```python
from build123d import *

# Parameters (mm, degrees)
F0_W     = 180
F0_H     = 40
F1_DEPTH = 22
F3_D     = 22
F3_DEPTH = 15
F3_TIP   = 6.6094668093
F5_D     = 11
F5_DEPTH = 12
F5_TIP   = 3.3047334047
F7_D     = 11
F7_DEPTH = 12
F7_TIP   = 3.3047334047
F9_D     = 11
F9_DEPTH = 12
F9_TIP   = 3.3047334047


with BuildPart() as f1:
    # F0 (on Top) → F1 (new body)
    with BuildSketch(Plane.XY):
        Rectangle(F0_W, F0_H)
    extrude(amount=-F1_DEPTH)

    # F3
    with Locations(Plane.XY):
        with Locations((0, 0)):
            Hole(F3_D / 2, depth=F3_DEPTH)
            with Locations((0, 0, -(F3_DEPTH + F3_TIP / 2))):  # 118° drill point
                Cone(0, F3_D / 2, F3_TIP, mode=Mode.SUBTRACT)

    # F5
    with Locations(Plane(origin=(-90, 0, 0), x_dir=(0, -1, 0), z_dir=(-1, 0, 0))):
        with Locations((0, -11)):
            Hole(F5_D / 2, depth=F5_DEPTH)
            with Locations((0, 0, -(F5_DEPTH + F5_TIP / 2))):  # 118° drill point
                Cone(0, F5_D / 2, F5_TIP, mode=Mode.SUBTRACT)

    # F7
    with Locations(Plane.YZ.offset(90)):
        with Locations((0, -11)):
            Hole(F7_D / 2, depth=F7_DEPTH)
            with Locations((0, 0, -(F7_DEPTH + F7_TIP / 2))):  # 118° drill point
                Cone(0, F7_D / 2, F7_TIP, mode=Mode.SUBTRACT)

    # F9
    with Locations(Plane(origin=(0, 20, 0), x_dir=(-1, 0, 0), z_dir=(0, 1, 0))):
        with Locations((-50, -11)):
            Hole(F9_D / 2, depth=F9_DEPTH)
            with Locations((0, 0, -(F9_DEPTH + F9_TIP / 2))):  # 118° drill point
                Cone(0, F9_D / 2, F9_TIP, mode=Mode.SUBTRACT)


solid = f1.part
```
Verification items for the finished model (mm, model axes). A direction names the side the tool comes from. Round coordinates to 2 decimals unless told otherwise and drop trailing zeros. Answer as a JSON object with one key per item and string values. Group by question number.
Q1. Mould release check, pull along Z, two halves, no side actions. Record for faces 1 (the cylindrical face through (-83.92, -1.19, -16.37)), 2 (the flat face through (-1, 0, -22)), 3 (the conical face through (49.12, 5.27, -11.37)), 4 (the flat face through (-1, 14, 0)): released by +Z, released by -Z, zero draft, split by the parting line, or undercut.
Q2. Tool access check on faces 5 (the cylindrical face through (44.505, 13.916, -10.758)), 6 (the cylindrical face through (83.92, 1.19, -16.37)), 7 (the flat face through (-1, 20, -11)), 8 (the cylindrical face through (2.38, -10.74, -7.6)), 9 (the flat face through (90, -5, -6)). Record the directions out of +Z, -Z, +X, -X, +Y, -Y that give a thin tool (end or side, any length) a straight path to the whole face; none if there is none.
Q3. Thickness scan on line 1 (Z direction, x = -87, y = 0); line 2 (Y direction, x = -84.5, z = -11); line 3 (X direction, y = 9, z = -4.5). Record the ranges inside material, lowest first.
Q4. Go/stop test with flat-tipped pins: pin 1 Ø1.5 at (y, z) = (4, -10.5) entering from -X; pin 2 Ø10 at (y, z) = (0, -11) entering from +X; pin 3 Ø10 at (y, z) = (0, -11) entering from -X. Record where each tip stops, or that it passes through.
Found:
{
 "1": {"face 1": "undercut", "face 2": "released by -Z", "face 3": "undercut", "face 4": "released by +Z"},
 "2": {"face 5": "+Y", "face 6": "+X", "face 7": "+Z, -Z, +X, -X, +Y", "face 8": "+Z", "face 9": "+Z, -Z, +X, +Y, -Y"},
 "3": {"line 1": "z = -22 to -16.5, -5.5 to 0", "line 2": "y = -20 to -5.5, 5.5 to 20", "line 3": "x = -90 to -6.32, 6.32 to 90"},
 "4": {"pin 1": "stops at x = -77.57", "pin 2": "stops at x = 77.7", "pin 3": "stops at x = -77.7"}
}
